Geometry: see drawing. Coordinates: mm, zero at the bounding-box minimum. A direction names the side the tool comes from. Give positions to 0.01 mm unless a question says otherwise; leave off trailing zeros. Order: outer loops, then holes, each group sorted by start corner. A loop starts at its lowest first (then second) coordinate and runs counter-clockwise, first axis right, second up. Notation, with made-up numbers: (66.25, 46.5) - (100.25, 46.5) arc R31 ccw to (100.25, 72.5) - close; hole circle Ø6 at (15.25, 28). An arc over 180 degrees is marked (long way). Write each question's results on one line, items separated by ' | '. Start each with the question number.
Item 1: Contact query for flat-ended pins moving along their axis: pin 1 Ø4 at (y, z) = (16, 8.5) entering from +X; pin 2 Ø0.6 at (x, y) = (48, 13.5) entering from -Z; pin 3 Ø2.5 at (x, y) = (12.75, 12.5) entering from +Z; pin 4 Ø6 at (x, y) = (34, 17.5) entering from -Z. Output: stop coordinate, or through.
Item 2: Line query: line 1 along X through (y, z) = (12, 16.25); line 2 along X through (y, z) = (6.25, 12.75); line 3 along Y through (x, z) = (39.25, 22.25). Output: solid intervals per line, ascending.
Item 3: Section B-B on z = 6. Output: boundary loops of the cut face in (x, y), and give its area (3 significant figures).
Item 4: Section A-A on x = 12.75. Output: boundary loops of the cut face in (y, z), and give its area (3 significant figures).
Item 5: Set-up query: the marked faces 1 and 2. Return all of +Z, -Z, +X, -X, +Y, -Y with unobstructed straight access to the full face (end or side cutting, diameter ignored); none if empty.
Item 6: Section C-C on y = 12.5. Output: boundary loops of the cut face in (x, z), and give its area (3 significant figures).
Item 7: Mould query, pull axis X, two halves, no side actions, for the marked faces 3, 4, 5 and 6. Classes: released by +X, released by -X, zero draft, split by the parting line, or undercut.
Item 8: Section D-D on y = 4.75. Output: boundary loops of the cut face in (x, z), and give its area (3 significant figures).
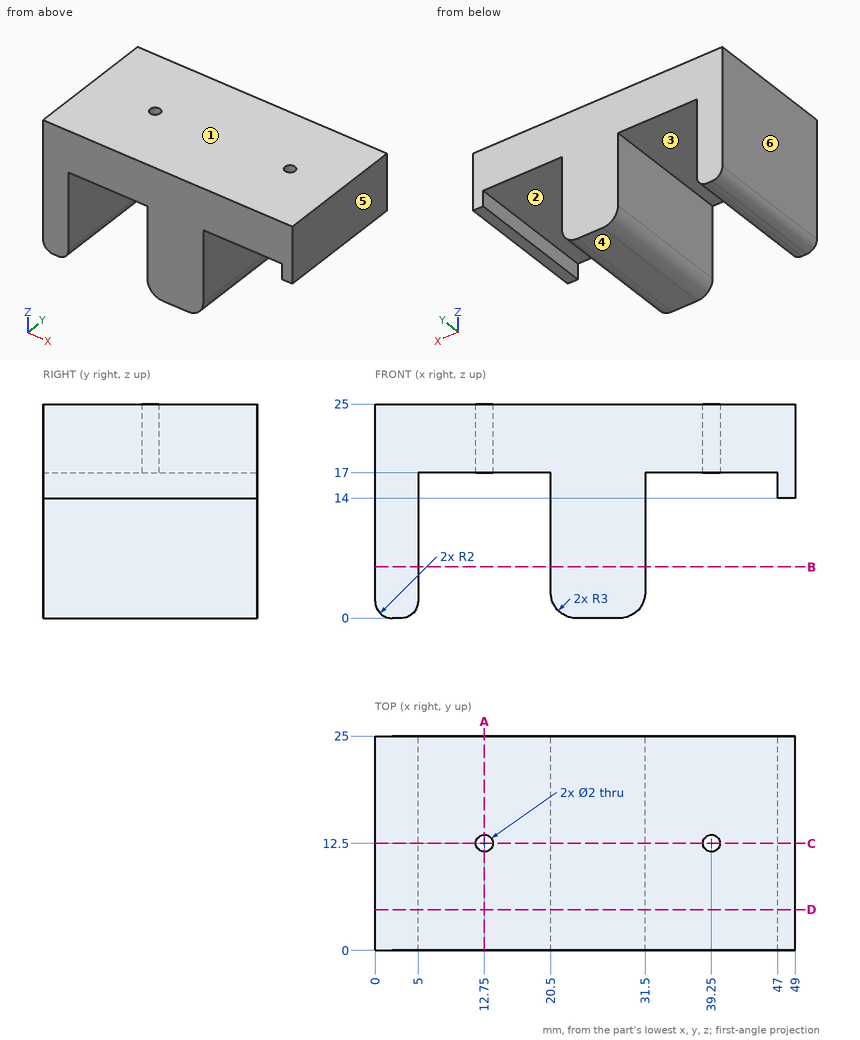
Evaluation:
1) pin 1: stops at x = 31.5 | pin 2: stops at z = 14 | pin 3: stops at z = 25 | pin 4: stops at z = 1.34
2) line 1: x = 0 to 5, 20.5 to 31.5, 47 to 49 | line 2: x = 0 to 5, 20.5 to 31.5 | line 3: y = 0 to 11.5, 13.5 to 25
3) outline: (0, 0) - (5, 0) - (5, 25) - (0, 25) - close; (20.5, 0) - (31.5, 0) - (31.5, 25) - (20.5, 25) - close | area: 400 mm^2
4) outline: (0, 17) - (11.5, 17) - (11.5, 25) - (0, 25) - close; (13.5, 17) - (25, 17) - (25, 25) - (13.5, 25) - close | area: 184 mm^2
5) face 1: +Z, +X, -X, +Y, -Y | face 2: -Z, +Y, -Y
6) outline: (0, 2) arc R2 ccw to (2, 0) - (3, 0) arc R2 ccw to (5, 2) - (5, 17) - (11.75, 17) - (11.75, 25) - (0, 25) - close; (13.75, 17) - (20.5, 17) - (20.5, 3) arc R3 ccw to (23.5, 0) - (28.5, 0) arc R3 ccw to (31.5, 3) - (31.5, 17) - (38.25, 17) - (38.25, 25) - (13.75, 25) - close; (40.25, 17) - (47, 17) - (47, 14) - (49, 14) - (49, 25) - (40.25, 25) - close | area: 632 mm^2
7) face 3: undercut | face 4: zero draft | face 5: released by +X | face 6: released by -X
8) outline: (0, 2) arc R2 ccw to (2, 0) - (3, 0) arc R2 ccw to (5, 2) - (5, 17) - (20.5, 17) - (20.5, 3) arc R3 ccw to (23.5, 0) - (28.5, 0) arc R3 ccw to (31.5, 3) - (31.5, 17) - (47, 17) - (47, 14) - (49, 14) - (49, 25) - (0, 25) - close | area: 664 mm^2
